Build history of the part. All positions in model axes, mm. A direction names the side the tool comes from. Give positions to 0.01 mm unless a question says otherwise; leave off trailing zeros. Order: outer loops, then holes, each group sorted by start corner. A loop starts at its lowest first (then second) coordinate and runs counter-clockwise, first axis right, second up. Notation, with made-up numbers: (73, 37) - (116, 37) arc R16 cw to (116, 62) - close; hole circle Ø6 at (-7, 24). An arc over 180 degrees is marked (long way). Answer in a Markdown table with one row per item.
```python
from build123d import *

# Parameters (mm, degrees)
SKETCH1_R           = 5
BOSS_EXTRUDE1_DEPTH = 14
SKETCH2_R           = 6
BOSS_EXTRUDE2_DEPTH = 10
SKETCH3_R           = 6.5
BOSS_EXTRUDE3_DEPTH = 26
SKETCH4_R           = 7
BOSS_EXTRUDE4_DEPTH = 12
SKETCH5_W           = 4
SKETCH5_H           = 20
CUT_EXTRUDE2_DEPTH  = 2


with BuildPart() as part:
    # Sketch1 → Boss-Extrude1 (new body)
    with BuildSketch(Plane(origin=(0, 0, 0), x_dir=(0, 1, 0), z_dir=(0, 0, 1))):
        with Locations(Location((0, 0, 0), (0, 0, 270))):
            Circle(SKETCH1_R)
    extrude(amount=BOSS_EXTRUDE1_DEPTH)

    # Sketch2 → Boss-Extrude2 (add)
    with BuildSketch(Plane.XY.offset(14)):
        Circle(SKETCH2_R)
    extrude(amount=BOSS_EXTRUDE2_DEPTH)

    # Sketch3 → Boss-Extrude3 (add)
    with BuildSketch(Plane.XY.offset(24)):
        with Locations(Location((0, 0, 0), (0, 0, 180))):
            Circle(SKETCH3_R)
    extrude(amount=BOSS_EXTRUDE3_DEPTH)

    # Sketch4 → Boss-Extrude4 (add)
    with BuildSketch(Plane.XY.offset(50)):
        Circle(SKETCH4_R)
    extrude(amount=BOSS_EXTRUDE4_DEPTH)

    # Mirror1: part across plane


with BuildPart() as part_1:
    add(part.part)
    add(part.part.mirror(Plane.XY.offset(62)))

    # Sketch5 → Cut-Extrude2 (cut)
    with BuildSketch(Plane(origin=(0, 7, 0), x_dir=(-1, 0, 0), z_dir=(0, 1, 0))):
        with Locations((0, 62)):
            Rectangle(SKETCH5_W, SKETCH5_H)
    extrude(amount=-CUT_EXTRUDE2_DEPTH, mode=Mode.SUBTRACT)


solid = part_1.part
```
1. Probe line 1 (Z direction, x = 1.75, y = 5.5); line 2 (X direction, y = 0.25, z = 109); line 3 (Z direction, x = -3.5, y = 4.5). List the from-to ranges inside material, lowest first.
Check result:
| item | result |
|---|---|
| line 1 | z = 14 to 52, 72 to 110 |
| line 2 | x = -5.99 to 5.99 |
| line 3 | z = 14 to 110 |
2. Cut at A-A on y = 0. Write the cut outline in (x, z), and give its area (3 significant figures).
Check result:
| item | result |
|---|---|
| outline | (-7, 50) - (-6.5, 50) - (-6.5, 24) - (-6, 24) - (-6, 14) - (-5, 14) - (-5, 0) - (5, 0) - (5, 14) - (6, 14) - (6, 24) - (6.5, 24) - (6.5, 50) - (7, 50) - (7, 74) - (6.5, 74) - (6.5, 100) - (6, 100) - (6, 110) - (5, 110) - (5, 124) - (-5, 124) - (-5, 110) - (-6, 110) - (-6, 100) - (-6.5, 100) - (-6.5, 74) - (-7, 74) - close |
| area | 1,530 mm² |
3. Two-plate mould, pull along Z, no slides. Class faces 1 (the face through (-6, 0, 105)), 2 (the face through (0, 6, 52)), 3 (the face through (-2, 6, 24)): +Z half, -Z half, draft (parallel to the pull), parting line (faces both ways), or undercut.
Check result:
| item | result |
|---|---|
| face 1 | draft |
| face 2 | undercut |
| face 3 | -Z half |
4. Which spindle directions (+Z, -Z, +X, -X, +Y, -Y) get a long thin tool onto all of the face, cutting with end or side? Do faces 4 (the face through (3.23, -6.21, 62.17)), 5 (the face through (0, 6, 72)), 6 (the face through (-4, 4, 110)), 7 (the face through (-4, 4, 14)). Say none if no direction does.
Check result:
| item | result |
|---|---|
| face 4 | +Z, -Z |
| face 5 | +Y |
| face 6 | +Z |
| face 7 | -Z |
5. Cut at D-D on z = 108. Write the cut outline in (x, y).
Check result:
| item | result |
|---|---|
| outline | circle Ø12 at (0, 0) |
6. Drop flat-ended pins along their axis: P1, Ø1.9, axis at y = 6, z = 58, coming from the +X side; P2, Ø1.2, axis at x = 0, z = 63, coming from the +Y side; P3, Ø2, axis at x = 0.5, z = 98.5, coming from the +Y side. Give the stop position or say it passes through.
Check result:
| item | result |
|---|---|
| P1 | stops at x = 4.85 |
| P2 | stops at y = 5 |
| P3 | stops at y = 6.5 |
7. Cut at C-C on z = 28. Write the cut outline in (x, y), and give its area (3 significant figures).
Check result:
| item | result |
|---|---|
| outline | circle Ø13 at (0, 0) |
| area | 133 mm² |
